from build123d import *

# Parameters (mm, degrees)
SKETCH1_R           = 18.8
SKETCH1_R_2         = 1
SKETCH1_W           = 28
SKETCH1_H           = 15
BOSS_EXTRUDE1_DEPTH = 4
CUT_EXTRUDE1_DEPTH  = 3
FILLET1_R           = 1


with BuildPart() as part:
    # Sketch1 → Boss-Extrude1 (new body)
    with BuildSketch(Plane.XY):
        Circle(SKETCH1_R)
        with Locations((-11.9, 11.985611511)):
            Circle(SKETCH1_R_2, mode=Mode.SUBTRACT)
        with Locations((11.9, 11.985611511)):
            Circle(SKETCH1_R_2, mode=Mode.SUBTRACT)
        with Locations((11.9, -11.985611511)):
            Circle(SKETCH1_R_2, mode=Mode.SUBTRACT)
        with Locations((-11.9, -11.985611511)):
            Circle(SKETCH1_R_2, mode=Mode.SUBTRACT)
        with Locations((0, 2)):
            Rectangle(SKETCH1_W, SKETCH1_H, mode=Mode.SUBTRACT)
    extrude(amount=BOSS_EXTRUDE1_DEPTH)

    # Sketch2 → Cut-Extrude1 (cut)
    with BuildSketch(Plane(origin=(0, 0, 0), x_dir=(-1, 0, 0), z_dir=(0, 0, -1))):
        Polygon((-14, 9.8), (-7, 9.8), (-7, 13.8), (7, 13.8), (7, 9.8), (14, 9.8), (14, -10.1), (7, -10.1), (7, -14.1), (-7, -14.1), (-7, -10.1), (-14, -10.1), align=None)
    extrude(amount=-CUT_EXTRUDE1_DEPTH, mode=Mode.SUBTRACT)

    # Fillet1
    fillet1_edges = [part.edges().sort_by_distance(p)[0] for p in [
        (7, 13.8, 1.5),
        (-7, 13.8, 1.5),
        (-7, -14.1, 1.5),
        (7, -14.1, 1.5),
    ]]
    fillet(fillet1_edges, radius=FILLET1_R)


solid = part.part
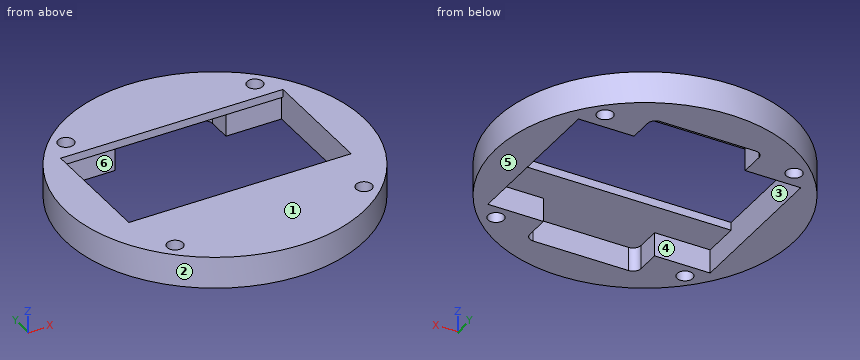
Verification items for the finished model (mm, model axes). Face numbers are marked on the shaded views. A direction names the side the tool comes from. Coordinates: 2 decimals unless noted, no trailing zeros. Write each loop counter-clockwise with the first axis right and the second up, starting at its lowest first coordinate (ties: lowest second). Pieces come first, ordered by that corner, then holes. Notation, with made-up numbers: M 49,-16.5 L 92,-16.5 A17 ccw 92,-3.5 Z; hole C -19,53.5 d2. An arc over 180 degrees is marked long. Use a Markdown table: item, result.
Q1. Sectioned sample at B-B, the plane x = -11.9. Record the boundary of the cut face in (y, z), plus the area to 3 significant figures.
Reply:
| item | result |
|---|---|
| outline | M -14.55,0 L -12.99,0 L -12.99,4 L -14.55,4 Z; M -10.99,0 L -10.1,0 L -10.1,3 L -5.5,3 L -5.5,4 L -10.99,4 Z; M 9.5,3 L 9.8,3 L 9.8,0 L 10.99,0 L 10.99,4 L 9.5,4 Z; M 12.99,0 L 14.55,0 L 14.55,4 L 12.99,4 Z |
| area | 25.7 mm² |
Q2. Sectioned sample at A-A, the plane y = 0. Record the boundary of the cut face in (x, z).
Reply:
| item | result |
|---|---|
| outline | M -18.8,0 L -14,0 L -14,4 L -18.8,4 Z; M 14,0 L 18.8,0 L 18.8,4 L 14,4 Z |
Q3. Thickness scan on line 1 (Y direction, x = -0.5, z = 0.9); line 2 (Y direction, x = -12, z = 3.2); line 3 (Y direction, x = 11.9, z = 2.8). Record the ranges inside material, lowest first.
Reply:
| item | result |
|---|---|
| line 1 | y = -18.79 to -14.1, 13.8 to 18.79 |
| line 2 | y = -14.47 to -12.98, -10.99 to -5.5, 9.5 to 10.99, 12.98 to 14.47 |
| line 3 | y = -14.55 to -12.99, -10.99 to -10.1, 9.8 to 10.99, 12.99 to 14.55 |
Q4. Sectioned sample at D-D, the plane x = 1.5. Record the boundary of the cut face in (y, z).
Reply:
| item | result |
|---|---|
| outline | M -18.74,0 L -14.1,0 L -14.1,3 L -5.5,3 L -5.5,4 L -18.74,4 Z; M 9.5,3 L 13.8,3 L 13.8,0 L 18.74,0 L 18.74,4 L 9.5,4 Z |
Q5. Set-up check for the marked faces 5 and 6: record each of +Z, -Z, +X, -X, +Y, -Y from which the full face is reachable in a straight line by a thin tool's end or side.
Reply:
| item | result |
|---|---|
| face 5 | -Z, +X, -X, +Y, -Y |
| face 6 | -Z |
Q6. Sectioned sample at C-C, the plane z = 3.55. Record the boundary of the cut face in (x, y).
Reply:
| item | result |
|---|---|
| outline | C 0,0 d37.6; hole M -14,-5.5 L 14,-5.5 L 14,9.5 L -14,9.5 Z; hole C -11.9,-11.99 d2; hole C -11.9,11.99 d2; hole C 11.9,-11.99 d2; hole C 11.9,11.99 d2 |
Q7. Go/stop test with flat-tipped pins: P1, Ø1.5, axis at x = -9, z = 1, coming from the +Y side; P2, Ø2, axis at y = -1.5, z = 2.5, coming from the -X side; P3, Ø1.5, axis at x = -12, z = 2, coming from the -Y side. Record where each tip stops, or that it passes through.
Reply:
| item | result |
|---|---|
| P1 | stops at y = 16.89 |
| P2 | stops at x = -18.79 |
| P3 | stops at y = -15.06 |
Q8. Draft check along Y on the marked faces 1, 2, 3 and 4. Enter one of: +Y half, -Y half, draft (parallel to the pull), parting line (faces both ways), or undercut.
Reply:
| item | result |
|---|---|
| face 1 | draft |
| face 2 | parting line |
| face 3 | undercut |
| face 4 | undercut |
